CAD build for the part. Positions are in the model's coordinates, mm. Give positions to 0.01 mm unless a question says otherwise; leave off trailing zeros. Write each loop counter-clockwise with the first axis right and the second up, starting at its lowest first coordinate (ties: lowest second). Pieces come first, ordered by that corner, then holes. Notation, with made-up numbers: (-1, -40) - (53, -40) arc R11 cw to (53, -32) - close; hole circle Ø1 at (68.25, 19). An arc over 180 degrees is marked (long way). Answer as a JSON object with one key per item and string values.
from build123d import *

# Parameters (mm, degrees)
SKETCH1_R           = 2.54
BOSS_EXTRUDE1_DEPTH = 0.79375


with BuildPart() as part:
    # Sketch1 → Boss-Extrude1 (new, symmetric)
    # profile 1 of 2: a face of its own
    with BuildSketch(Plane.XY):
        with BuildLine():
            Line((0, 10.938896076), (0, 12.7))
            Line((0, 12.7), (-7.260771792, 12.7))
            ThreePointArc((-7.260771792, 12.7), (-25.4, 5.08), (-43.539228208, 12.7))
            Line((-43.539228208, 12.7), (-58.060771792, 12.7))
            ThreePointArc((-58.060771792, 12.7), (-76.2, 5.08), (-94.339228208, 12.7))
            Line((-94.339228208, 12.7), (-101.6, 12.7))
            Line((-101.6, 12.7), (-101.6, 0))
            Line((-101.6, 0), (0, 0))
            Line((0, 0), (0, 5.858896076))
            ThreePointArc((0, 5.858896076), (-2.54, 8.398896076), (0, 10.938896076))
        make_face()
        with Locations((-96.562042846, 8.398896076)):
            Circle(SKETCH1_R, mode=Mode.SUBTRACT)
        with Locations((-50.984733006, 8.398896076)):
            Circle(SKETCH1_R, mode=Mode.SUBTRACT)
    # profile 2 of 2: a face of its own
    with BuildSketch(Plane.XY):
        with BuildLine():
            Line((7.260771792, 12.7), (0, 12.7))
            Line((0, 12.7), (0, 10.938896076))
            ThreePointArc((0, 10.938896076), (1.796051224, 10.1949473), (2.54, 8.398896076))
            ThreePointArc((2.54, 8.398896076), (1.796051224, 6.602844851), (0, 5.858896076))
            Line((0, 5.858896076), (0, 0))
            Line((0, 0), (101.6, 0))
            Line((101.6, 0), (101.6, 12.7))
            Line((101.6, 12.7), (94.339228208, 12.7))
            ThreePointArc((94.339228208, 12.7), (76.2, 5.08), (58.060771792, 12.7))
            Line((58.060771792, 12.7), (43.539228208, 12.7))
            ThreePointArc((43.539228208, 12.7), (25.4, 5.08), (7.260771792, 12.7))
        make_face()
        with Locations((50.984733006, 8.398896076)):
            Circle(SKETCH1_R, mode=Mode.SUBTRACT)
        with Locations((96.562042846, 8.398896076)):
            Circle(SKETCH1_R, mode=Mode.SUBTRACT)
    extrude(amount=BOSS_EXTRUDE1_DEPTH, both=True)


solid = part.part
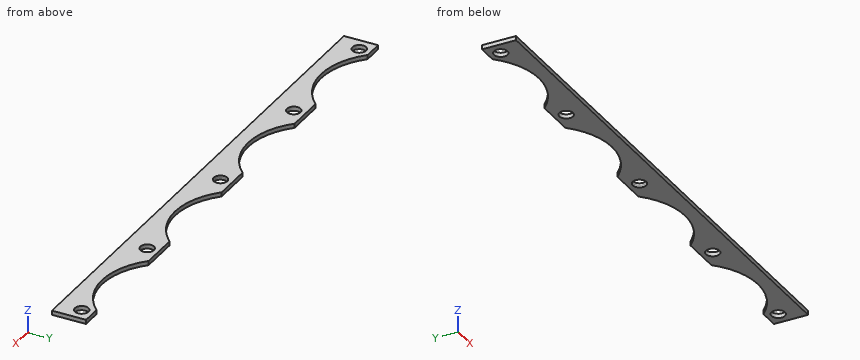
(1) Saw through at B-B, the plane x = 69. Give the cut face in (y, z).
Answer key:
{"outline": "(0, -0.79) - (6.12, -0.79) - (6.12, 0.79) - (0, 0.79) - close"}
(2) Saw through at A-A, the plane x = 36. Give the cut face in (y, z).
Answer key:
{"outline": "(0, -0.79) - (7.4, -0.79) - (7.4, 0.79) - (0, 0.79) - close"}
(3) Probe L1, parallel to X at y = 11.5, z = -0.55; L2, parallel to X at y = 11.25, z = 0.35; L3, parallel to Y at x = 1, z = 0.6. List the from-to ranges inside material, lowest first. Write a range as [from, to].
Answer key:
{"L1": "x = [-101.6, -93.08], [-59.32, -42.28], [-8.52, 8.52], [42.28, 59.32], [93.08, 101.6]", "L2": "x = [-101.6, -92.79], [-59.61, -41.99], [-8.81, 8.81], [41.99, 59.61], [92.79, 101.6]", "L3": "y = [0, 6.06], [10.73, 12.7]"}
